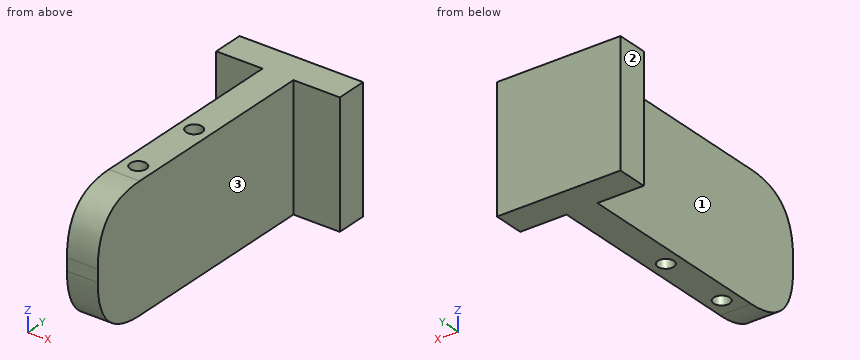
```python
from build123d import *

# Parameters (mm, degrees)
SKETCH_1_W           = 20
SKETCH_1_H           = 20
EXTRUDE_1_DEPTH      = 5
SKETCH_2_W           = 5
SKETCH_2_H           = 20
EXTRUDE_2_DEPTH      = 35
F_1_0MM_1_AT_2_COUNT = 2
F_1_0MM_1_AT_2_PITCH = 12
SKETCH_5_W           = 5
SKETCH_5_H           = 20
EXTRUDE_3_DEPTH      = 7
FILLET_1_SIZE        = 9


with BuildPart() as part:
    # 草圖1 → 填料-伸長1 (new body)
    with BuildSketch(Plane(origin=(0, 0, 0), x_dir=(1, 0, 0), z_dir=(0, 1, 0))):
        Rectangle(SKETCH_1_W, SKETCH_1_H)
    extrude(amount=EXTRUDE_1_DEPTH)

    # 草圖2 → 填料-伸長2 (add)
    with BuildSketch(Plane.XZ):
        Rectangle(SKETCH_2_W, SKETCH_2_H)
    extrude(amount=EXTRUDE_2_DEPTH)

    # 草圖4 → Ø1.0mm 定位孔1 (revolve, cut)
    with BuildSketch(Plane(origin=(0, -18, 10), x_dir=(0, -1, 0), z_dir=(1, 0, 0))):
        Polygon((0, 0), (0, 7.281118805), (1.3, 6.5), (1.3, 0), align=None)
    f_1_0mm_1 = revolve(axis=Axis((0, -18, 16.35), (0, 0, -1)), mode=Mode.SUBTRACT)

    # Ø1.0mm 定位孔1 at 2: Ø1.0mm 定位孔1 ×2
    with Locations(*[(0, -i * F_1_0MM_1_AT_2_PITCH, 0) for i in range(1, F_1_0MM_1_AT_2_COUNT)]):
        add(f_1_0mm_1, mode=Mode.SUBTRACT)

    # 鏡射1: Ø1.0mm 定位孔1 across plane
    add(f_1_0mm_1.mirror(Plane.XY), mode=Mode.SUBTRACT)

    # 鏡射1 copy 1 sketch → 鏡射1 copy 1 (revolve, cut)
    with BuildSketch(Plane(origin=(0, -30, -10), x_dir=(0, -1, 0), z_dir=(1, 0, 0))):
        Polygon((0, 0), (0, -7.281118805), (1.3, -6.5), (1.3, 0), align=None)
    revolve(axis=Axis((0, -30, -16.35), (0, 0, -1)), mode=Mode.SUBTRACT)

    # 草圖5 → 填料-伸長3 (add)
    with BuildSketch(Plane.XZ.offset(35)):
        Rectangle(SKETCH_5_W, SKETCH_5_H)
    extrude(amount=EXTRUDE_3_DEPTH)

    # 圓角1
    # a fillet whose section is not a circle: 9 mm, written as the material it takes off along each edge
    with BuildSketch(Plane(origin=(-25, -42, 10), x_dir=(0, 1, 0), z_dir=(1, 0, 0)), Plane(origin=(25, -42, -10), x_dir=(0, 1, 0), z_dir=(-1, 0, 0))) as fillet_1_piece_1:
        with BuildLine():
            Bezier((FILLET_1_SIZE, 0), (0, 0), (0, -FILLET_1_SIZE), weights=[1, 1, 1])
            Line((0, -FILLET_1_SIZE), (0, 0))
            Line((0, 0), (FILLET_1_SIZE, 0))
        make_face()
    extrude(amount=50, mode=Mode.SUBTRACT)


solid = part.part
```
Can you work these out from the model? Positions are in its coordinate system, mm. Face numbers are marked on the shaded views. A direction names the side the tool comes from. Round coordinates to 2 decimals unless told otherwise and drop trailing zeros. Loops run counter-clockwise (first coordinate to the right, second up) from the corner with the lowest first, then second, coordinate; pieces in that order, holes last.
Item 1: Please list where these lines run through material, in increasing order: L1, parallel to X at y = -30, z = -6; L2, parallel to Y at x = 0, z = -6.75; L3, parallel to Y at x = 0, z = -8.5.
Item 2: Suppose I cut it at A-A, the plane z = -7.75. State how many separate pieces and enclosed holes the cut face has, then the cut area to 3 significant figures.
Item 3: Will these pins go through, and if not, where does the flat tip stop? pin 1 Ø2 at (x, z) = (-7.5, -0.5) entering from -Y; pin 2 Ø2.5 at (x, y) = (0, -18) entering from -Z; pin 3 Ø1.5 at (y, z) = (-29, -4) entering from +X.
Item 4: Which directions (+Z, -Z, +X, -X, +Y, -Y) give clear straight access to the entire face, cutting with the end or side of a thin tool? Please do the marked faces 1, 2 and 3.
Item 5: Suppose I cut it at C-C, the plane y = -13.5. Write out the boundary of the cut face in (x, z), then the cut area to 3 significant figures.
Item 6: Suppose I cut it at B-B, the plane x = 6. Write out the boundary of the cut face in (y, z).
Reported:
1. L1: x = -2.5 to -1.3, 1.3 to 2.5
1. L2: y = -40.57 to -31.3, -28.7 to -19.3, -16.7 to 5
1. L3: y = -38.85 to -31.3, -28.7 to -19.3, -16.7 to 5
2. separate pieces: 1
2. enclosed holes: 2
2. area: 288 mm2
3. pin 1: stops at y = 0
3. pin 2: stops at z = -3.47
3. pin 3: stops at x = 2.5
4. face 1: +Z, -Z, -X, -Y
4. face 2: +Z, -Z, -X, +Y, -Y
4. face 3: +Z, -Z, +X, -Y
5. outline: (-2.5, -10) - (2.5, -10) - (2.5, 10) - (-2.5, 10) - close
5. area: 100 mm2
6. outline: (0, -10) - (5, -10) - (5, 10) - (0, 10) - close
